Here's how the part is built. I have some questions about the finished solid (model axes, mm). A direction names the side the tool comes from. Coordinates: 2 decimals unless noted, no trailing zeros. Order: outer loops, then holes, each group sorted by start corner. A loop starts at its lowest first (then second) coordinate and runs counter-clockwise, first axis right, second up.
Autodesk Inventor part; units mm, degrees
ref_plane "YZ Plane" through (0, 0, 0) normal (1, 0, 0) x (0, 1, 0)
ref_plane "XZ Plane" through (0, 0, 0) normal (0, 1, 0) x (-1, 0, 0)
ref_plane "XY Plane" through (0, 0, 0) normal (0, 0, 1) x (1, 0, 0)
sketch "Sketch1" plane through (0, 0, 0) normal (0, 1, 0) x (-1, 0, 0)
  line L0 (13.925, -3.65) -> (-13.925, -3.65)
  line L1 (-13.925, -3.65) -> (-13.925, 3.65)
  line L2 (-13.925, 3.65) -> (13.925, 3.65)
  line L3 (13.925, 3.65) -> (13.925, -3.65)
  line L4 (13.925, -3.65) -> (-13.925, 3.65) construction
  line L5 (-13.925, -3.65) -> (13.925, 3.65) construction
  line L6 (11.725, -1.25) -> (-11.725, -1.25)
  line L7 (-11.725, -1.25) -> (-11.725, 1.25)
  line L8 (-11.725, 1.25) -> (11.725, 1.25)
  line L9 (11.725, 1.25) -> (11.725, -1.25)
  line L10 (11.725, -1.25) -> (-11.725, 1.25) construction
  line L11 (-11.725, -1.25) -> (11.725, 1.25) construction
  line L12 (11.725, -1.25) -> (11.725, -3.65) construction
  line L13 (11.725, 1.25) -> (11.725, 3.65) construction
  line L14 (11.725, -1.25) -> (13.925, -1.25) construction
  line L15 (-11.725, -1.25) -> (-13.925, -1.25) construction
  point P0 (0, 0)
  point P1 (0, 0)
  point P2 (0, 0)
  point P3 (0, 0)
  dimension "d0" = 27.85
  dimension "d1" = 7.3
  dimension "d2" = 2.4
  dimension "d3" = 2.4
  dimension "d4" = 2.5
  dimension "d5" = 2.2
  dimension "d6" = 23.45
sketch "Sketch2" plane through (0, 0, 0) normal (0, 1, 0) x (-1, 0, 0)
  line L0 (17.5, 8) -> (-17.5, 8)
  line L1 (-17.5, 8) -> (-17.5, -8)
  line L2 (-17.5, -8) -> (17.5, -8)
  line L3 (17.5, -8) -> (17.5, 8)
  line L4 (17.5, 8) -> (-17.5, -8) construction
  point P0 (0, 0)
  point P1 (0, 0)
  dimension "d7" = 35
  dimension "d8" = 16
extrude "Extrusion1" add sketch "Sketch2" against normal blind 4
sketch "Sketch5" plane through (0, 0, 0) normal (0, 1, 0) x (1, 0, 0)
  line L0 (-12.925, -2.45) -> (12.925, -2.45)
  line L1 (12.925, -2.45) -> (12.925, 2.45)
  line L2 (12.925, 2.45) -> (-12.925, 2.45)
  line L3 (-12.925, 2.45) -> (-12.925, -2.45)
  line L4 (-12.925, -2.45) -> (12.925, 2.45) construction
  line L5 (11.725, -1.25) -> (-11.725, -1.25) construction
  line L6 (-11.725, 1.25) -> (11.725, 1.25) construction
  line L7 (24.5, 0) -> (-24.5, 0) construction
  line L8 (0, 11.2) -> (0, -11.2) construction
  point P0 (0, 0)
  point P1 (0, 0)
  dimension "d11" = 1.2
  dimension "d12" = 1.2
extrude "Extrusion2" cut sketch "Sketch5" against normal blind 2
fillet "Fillet1" radius 1.2 4 edges at (12.925, -1, 2.45) (-12.925, -1, 2.45) (-12.925, -1, -2.45) (12.925, -1, -2.45)
sketch "Sketch6" plane through (0, 0, 0) normal (0, 1, 0) x (1, 0, 0)
  arc A0 (12.925, 1.25) -> (11.725, 2.45) centre (11.725, 1.25) ccw
  line L0 (-11.725, 2.45) -> (11.725, 2.45)
  arc A1 (-11.725, 2.45) -> (-12.925, 1.25) centre (-11.725, 1.25) ccw
  line L1 (-12.925, -1.25) -> (-12.925, 1.25)
  arc A2 (-12.925, -1.25) -> (-11.725, -2.45) centre (-11.725, -1.25) ccw
  line L2 (11.725, -2.45) -> (-11.725, -2.45)
  arc A3 (11.725, -2.45) -> (12.925, -1.25) centre (11.725, -1.25) ccw
  line L3 (12.925, 1.25) -> (12.925, -1.25)
  arc A4 (14.425, 1.25) -> (11.725, 3.95) centre (11.725, 1.25) ccw
  line L4 (14.425, 1.25) -> (14.425, -1.25)
  arc A5 (11.725, -3.95) -> (14.425, -1.25) centre (11.725, -1.25) ccw
  line L5 (11.725, -3.95) -> (-11.725, -3.95)
  arc A6 (-14.425, -1.25) -> (-11.725, -3.95) centre (-11.725, -1.25) ccw
  line L6 (-14.425, -1.25) -> (-14.425, 1.25)
  arc A7 (-11.725, 3.95) -> (-14.425, 1.25) centre (-11.725, 1.25) ccw
  line L7 (-11.725, 3.95) -> (11.725, 3.95)
  line L8 (-15.625, 1.25) -> (-15.625, -1.25)
  arc A8 (-15.625, -1.25) -> (-11.725, -5.15) centre (-11.725, -1.25) ccw
  line L9 (-11.725, -5.15) -> (11.725, -5.15)
  arc A9 (11.725, -5.15) -> (15.625, -1.25) centre (11.725, -1.25) ccw
  line L10 (15.625, -1.25) -> (15.625, 1.25)
  arc A10 (15.625, 1.25) -> (11.725, 5.15) centre (11.725, 1.25) ccw
  line L11 (11.725, 5.15) -> (-11.725, 5.15)
  arc A11 (-11.725, 5.15) -> (-15.625, 1.25) centre (-11.725, 1.25) ccw
  point P0 (0, 0)
  dimension "d16" = 1.5
  dimension "d17" = 1.2
extrude "Extrusion3" cut sketch "Sketch6" against normal blind 0.6 contours A11 L11 A10 L10 A9 L9 A8 L8
sketch "Sketch7" plane through (0, 0, 0) normal (0, 1, 0) x (1, 0, 0)
  line L0 (-29.5, -10) -> (29.5, -10)
  line L1 (29.5, -10) -> (29.5, 10)
  line L2 (29.5, 10) -> (-29.5, 10)
  line L3 (-29.5, 10) -> (-29.5, -10)
  line L4 (-41.3, 0) -> (41.3, 0) construction
  line L5 (0, 14) -> (0, -14) construction
  line L6 (-17.5, 8) -> (-17.5, -8) construction
  line L7 (17.5, 8) -> (-17.5, 8) construction
  point P0 (0, 0)
  dimension "d20" = 12
  dimension "d21" = 2
equation "\"d12\" = d11"
properties part number "Capping_Insert"
Q1. For faces 4 (the flat face through (0, -4, 0)), 5 (the cylindrical face through (13.613, -0.296, 3.18)), which set-ups out of +Z, -Z, +X, -X, +Y, -Y let a thin tool reach every point of the face, with its end or its side?
Q2. If we section it at A-A on y = -1.5: Write out the boundary of the cut face in (x, z) (3 decimals).
Q3. Will this pin go through, and if not, where does the flat tip stop? pin 1 (1.5 mm diameter, centred on x = 3.5, z = 0.5, fed in from +Y).
Q4. We'd pull the mould along X, two halves only. Please class faces 1 (the flat face through (17.5, -2, 0)), 2 (the flat face through (0, -2, -8)), 3 (the cylindrical face through (12.58, -1.01, 2.09)): pulls with the +X half, pulls with the -X half, needs draft (parallel to the pull), parting line crosses it, or undercut.
Q5. If we section it at B-B on x = 6: Write out the boundary of the cut face in (y, z).
Q6. If we section it at C-C on z = -2: Write out the boundary of the cut face in (x, y).
Q7. I need wall thicknesses on L1, parallel to Z at x = 6, y = -0.7; L2, parallel to X at y = -0.35, z = 0.5 (3 decimals); L3, parallel to Y at x = 5.5, z = -5. Which ranges of each line are inside material? Lowest first, please.
Reply:
1. face 4: +Z, -Z, +X, -X, -Y
1. face 5: +Y
2. outline: (-17.5, -8) - (17.5, -8) - (17.5, 8) - (-17.5, 8) - close; hole (-12.925, -1.25) arc R1.2 ccw to (-11.725, -2.45) - (11.725, -2.45) arc R1.2 ccw to (12.925, -1.25) - (12.925, 1.25) arc R1.2 ccw to (11.725, 2.45) - (-11.725, 2.45) arc R1.2 ccw to (-12.925, 1.25) - close
3. pin 1: stops at y = -2
4. face 1: pulls with the +X half
4. face 2: needs draft
4. face 3: undercut
5. outline: (-4, -8) - (0, -8) - (0, -5.15) - (-0.6, -5.15) - (-0.6, -3.95) - (0, -3.95) - (0, -2.45) - (-2, -2.45) - (-2, 2.45) - (0, 2.45) - (0, 3.95) - (-0.6, 3.95) - (-0.6, 5.15) - (0, 5.15) - (0, 8) - (-4, 8) - close
6. outline: (-17.5, -4) - (17.5, -4) - (17.5, 0) - (15.55, 0) - (15.55, -0.6) - (14.32, -0.6) - (14.32, 0) - (12.66, 0) - (12.66, -2) - (-12.66, -2) - (-12.66, 0) - (-14.32, 0) - (-14.32, -0.6) - (-15.55, -0.6) - (-15.55, 0) - (-17.5, 0) - close
7. L1: z = -8 to -2.45, 2.45 to 8
7. L2: x = -17.5 to -15.625, -14.425 to -12.925, 12.925 to 14.425, 15.625 to 17.5
7. L3: y = -4 to -0.6
